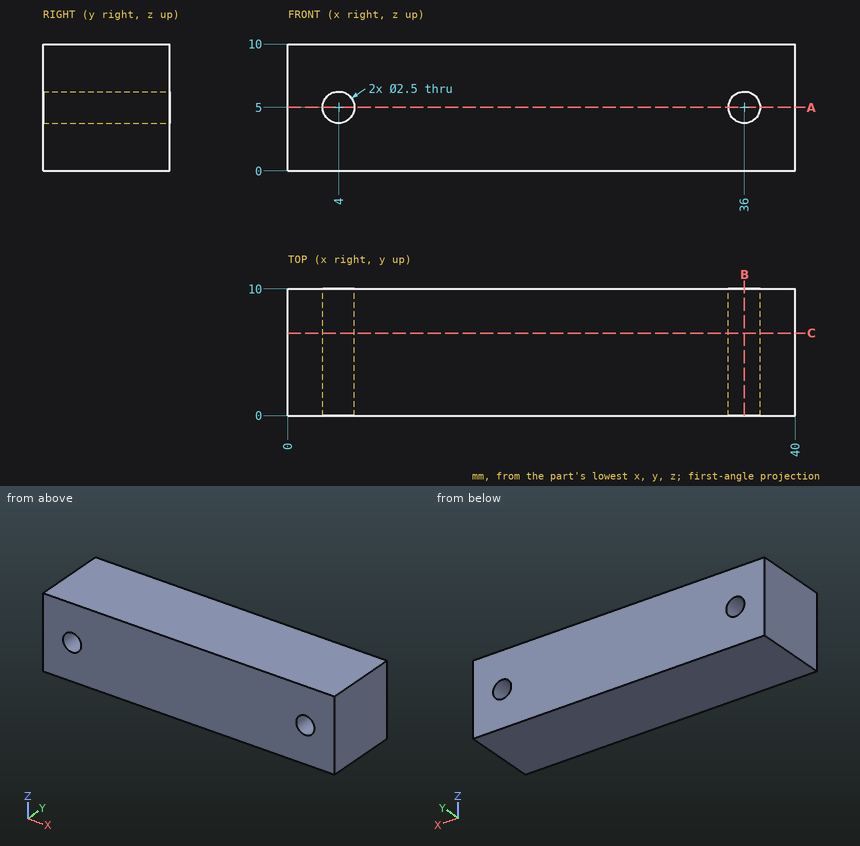
The figure shows three views and two pictorial views of one solid part (mm, origin at its lowest corner). Answer the questions. Give positions to 0.01 mm unless a question says otherwise; leave off trailing zeros. Write each loop counter-clockwise with the first axis right and the second up, starting at its lowest first coordinate (ties: lowest second). Pieces come first, ordered by that corner, then holes. Notation, with made-up numbers: (-13, 20.5) - (23, 20.5) arc R21 ccw to (23, 32.5) - close; hole circle Ø3 at (40, 67). An arc over 180 degrees is marked (long way). Use one line per item in the form item = value. Start each with the question number.
1) Consider line 1 along X through (y, z) = (4.5, 5); line 2 along Z through (x, y) = (36, 2.75); line 3 along X through (y, z) = (0.5, 4.5). Determine where each line is inside the solid, lowest interval first. Write a range as from..to.
2) Find section A-A on z = 5. Determine the outline of the cut face in (x, y).
3) A flat-ended cylindrical pin translates along its axis: pin 1 Ø1.5 at (x, z) = (36, 5) entering from -Y. Find the tip coordinate at first contact, or state that the pin passes through.
4) Find section C-C on y = 6.5. Determine the outline of the cut face in (x, z), plus the area to 3 significant figures.
5) Find section B-B on x = 36. Determine the outline of the cut face in (y, z).
Geometry results:
q1.line_1 = 0..2.75, 5.25..34.75, 37.25..40
q1.line_2 = 0..3.75, 6.25..10
q1.line_3 = 0..2.85, 5.15..34.85, 37.15..40
q2.outline = (0, 0) - (2.75, 0) - (2.75, 10) - (0, 10) - close; (5.25, 0) - (34.75, 0) - (34.75, 10) - (5.25, 10) - close; (37.25, 0) - (40, 0) - (40, 10) - (37.25, 10) - close
q3.pin_1 = through
q4.outline = (0, 0) - (40, 0) - (40, 10) - (0, 10) - close; hole circle Ø2.5 at (4, 5); hole circle Ø2.5 at (36, 5)
q4.area = 390 mm2
q5.outline = (0, 0) - (10, 0) - (10, 3.75) - (0, 3.75) - close; (0, 6.25) - (10, 6.25) - (10, 10) - (0, 10) - close
